Can you work these out from the model? Positions are in its coordinate system, mm. A direction names the side the tool comes from. Give positions to 0.01 mm unless a question says otherwise; leave off trailing zeros. Loops run counter-clockwise (first coordinate to the right, second up) from the corner with the lowest first, then second, coordinate; pieces in that order, holes last. Notation, with made-up numbers: M 62.25,73 L 76.25,73 A18 ccw 76.25,82 Z; hole C -35,61 d8. An arc over 180 degrees is marked long. Put each result on its own line as item: value. Start each with the question number.
1) Imagine slicing it at B-B (y = -0.5). Write out the boundary of the cut face in (x, z), then the cut area to 3 significant figures.
2) Imagine slicing it at D-D (z = 8.5). Write out the boundary of the cut face in (x, y), then the cut area to 3 significant figures.
3) For faces 1 (the flat face through (-6.858, -1, -3)), 2 (the flat face through (0, -1.778, 5)), which set-ups out of +Z, -Z, +X, -X, +Y, -Y let a thin tool reach every point of the face, with its end or its side?
4) Please list where these lines run through material, in increasing order: line 1 along X through (y, z) = (-1.25, -7.5); line 2 along Z through (x, y) = (-1.5, -1.7); line 3 along Y through (x, z) = (11, 9.75). Write a range as from..to.
5) Imagine slicing it at A-A (z = -8.25). Write out the boundary of the cut face in (x, y), then the cut area to 3 significant figures.
6) For P1, Ø0.9, axis at x = 0, y = -1, coming from the -Z side; P2, Ø11, axis at x = 0, z = -3.5, coming from the +Y side; P3, Ø2, axis at x = 9, z = 4.5, coming from the +Y side, each with a flat end and sliding along its axis, tell me the tip position at first contact or that it passes through.
7) Imagine slicing it at C-C (x = 1.5). Write out the boundary of the cut face in (y, z), then the cut area to 3 significant figures.
from build123d import *

# Parameters (mm, degrees)
F1_DEPTH = 1.778
F3_DEPTH = 6.35
F4_R     = 0.25399


# Not quite as in the source:
# - a fillet or chamfer is up to 0.001 mm smaller than in the source, because OpenCascade refuses the exact size


with BuildPart() as f1:
    # F0 (on Front) → F1 (new body)
    with BuildSketch(Plane.XZ):
        Polygon((-6.858, -10.8697404989), (-6.858, 4.3702595011), (0, 4.3702595011), (6.858, 4.3702595011), (6.858, -10.8697404989), (13.208, -10.8697404989), (13.208, 10.7202595011), (-13.208, 10.7202595011), (-13.208, -10.8697404989), align=None)
    extrude(amount=F1_DEPTH)

    # F2 (on Right) → F3 (join, symmetric)
    with BuildSketch(Plane.YZ):
        with BuildLine():
            ThreePointArc((0.254, 10.3265595011), (0.1849893869, 10.5608220088), (0, 10.7202595011))
            Line((0, 10.7202595011), (0, 10.3265595011))
            Line((0, 10.3265595011), (0.254, 10.3265595011))
        make_face()
        with BuildLine():
            Line((0.254, 10.3265595011), (0, 10.3265595011))
            Line((0, 10.3265595011), (0, 9.9328595011))
            ThreePointArc((0, 9.9328595011), (0.1849893869, 10.0922969934), (0.254, 10.3265595011))
        make_face()
    extrude(amount=F3_DEPTH, both=True)

    # F4 (radius 0.254 in the source; OpenCascade refuses exactly that, so slightly less here)
    f4_edges = [f1.edges().sort_by_distance(p)[0] for p in [
        (-6.35, 0.254, 10.32656),
        (6.35, 0.254, 10.32656),
    ]]
    fillet(f4_edges, radius=F4_R)


solid = f1.part
Recorded:
1. outline: M -13.21,-10.87 L -6.86,-10.87 L -6.86,4.37 L 6.86,4.37 L 6.86,-10.87 L 13.21,-10.87 L 13.21,10.72 L -13.21,10.72 Z
1. area: 361 mm²
2. outline: M -13.21,-1.78 L 13.21,-1.78 L 13.21,0 L -13.21,0 Z
2. area: 47.0 mm²
3. face 1: -Z, +Y, -Y
3. face 2: +Z, -Z, +X, -X, -Y
4. line 1: -13.21..-6.86, 6.86..13.21
4. line 2: 4.37..10.72
4. line 3: -1.78..0
5. outline: M -13.21,-1.78 L -6.86,-1.78 L -6.86,0 L -13.21,0 Z; M 6.86,-1.78 L 13.21,-1.78 L 13.21,0 L 6.86,0 Z
5. area: 22.6 mm²
6. P1: z = 4.37
6. P2: through
6. P3: y = 0
7. outline: M -1.78,4.37 L 0,4.37 L 0,9.93 A0.43 ccw 0,10.72 L -1.78,10.72 Z
7. area: 11.4 mm²
